from build123d import *

# Parameters (mm, degrees)
F1_DEPTH = 25
F2_R     = 10


with BuildPart() as f1:
    # F0 (on Front) → F1 (new body)
    with BuildSketch(Plane.XZ):
        Polygon((-26.120773, 31.526426), (-26.120773, -33.473574), (12.333255, -33.473574), (32.812056, -19.134163), (23.879227, 31.526426), align=None)
    extrude(amount=F1_DEPTH)

    # F2
    f2_edges = [f1.edges().sort_by_distance(p)[0] for p in [
        (23.879227, -12.5, 31.526426),
        (32.812056, -12.5, -19.134163),
        (-26.120773, -12.5, 31.526426),
        (-26.120773, -12.5, -33.473574),
        (28.345642, -25, 6.196132),
        (-1.120773, -25, 31.526426),
        (-26.120773, -25, -0.973574),
        (-6.893759, -25, -33.473574),
        (22.572655, -25, -26.303868),
        (28.345642, 0, 6.196132),
        (-1.120773, 0, 31.526426),
        (-26.120773, 0, -0.973574),
        (-6.893759, 0, -33.473574),
        (22.572655, 0, -26.303868),
    ]]
    fillet(f2_edges, radius=F2_R)


solid = f1.part
Could you check a few things on this model? Use its own coordinates, in mm. Coordinates: 2 decimals unless noted, no trailing zeros. Write each loop counter-clockwise with the first axis right and the second up, starting at its lowest first coordinate (ties: lowest second). Pieces come first, ordered by that corner, then holes. Notation, with made-up numbers: (9.25, 85.25) - (19.25, 85.25) arc R8 ccw to (19.25, 96.25) - close; hole circle Ø5 at (60, -5). An arc over 180 degrees is marked (long way). Put each result on its own line as item: value. Start each with the question number.
Q1. Thinking about a two-plate mould opening in X: for faces 1 (the flat face through (3, -25, -1)), 2 (the cylindrical face through (-23.27, -3.01, -1.29)), 3 (the flat face through (19.857, -12.465, -28.206)), which applies, pulls with the +X half, pulls with the -X half, needs draft (parallel to the pull), parting line crosses it, or undercut?
Q2. I want a section at B-B on y = -12. Write out the boundary of the cut face in (x, z).
Q3. I want a section at A-A on x = -3. Write out the boundary of the cut face in (y, z).
Q4. I want a section at C-C on z = 27.5. Write out the boundary of the cut face in (x, y), plus the area to 3 significant figures.
Q5. I'm going to push flat-ended pins straight in: P1, Ø6, axis at y = -6, z = 13.5, coming from the +X side; P2, Ø1.5, axis at y = -19, z = 14, coming from the -X side; P3, Ø1, axis at x = 24.5, y = -3.5, coming from the -Z side. Where does each tip first touch, or does it pass through?
Q6. Please list where these lines run through material, in increasing order: L1, parallel to X at y = -21, z = -1.5; L2, parallel to X at y = -11.25, z = -28; L3, parallel to Y at x = 1.5, z = 26.5.
Q7. I want a section at D-D on y = -5.75. Write out the boundary of the cut face in (x, z), plus the area to 3 significant figures.
Checks:
1. face 1: needs draft
1. face 2: pulls with the -X half
1. face 3: pulls with the +X half
2. outline: (-26.12, -23.47) arc R10 ccw to (-16.12, -33.47) - (12.33, -33.47) - (27.59, -22.79) arc R10 ccw to (31.71, -12.86) - (25.34, 23.26) arc R10 ccw to (15.49, 31.53) - (-16.12, 31.53) arc R10 ccw to (-26.12, 21.53) - close
3. outline: (-25, -23.47) arc R10 ccw to (-15, -33.47) - (-10, -33.47) arc R10 ccw to (0, -23.47) - (0, 21.53) arc R10 ccw to (-10, 31.53) - (-15, 31.53) arc R10 ccw to (-25, 21.53) - close
4. outline: (-24.14, -15) arc R8.02 ccw to (-16.12, -23.02) - (15.49, -23.02) arc R8.02 ccw to (23.51, -15) - (23.51, -10) arc R8.02 ccw to (15.49, -1.98) - (-16.12, -1.98) arc R8.02 ccw to (-24.14, -10) - close
4. area: 947 mm²
5. P1: x = 27.25
5. P2: x = -25.58
5. P3: z = -22.63
6. L1: -24.12 to 27.67
6. L2: -25.04 to 20.15
6. L3: -23.68 to -1.32
7. outline: (-25.17, -23.47) arc R9.05 ccw to (-16.12, -32.53) - (12.03, -32.53) - (27.05, -22.01) arc R9.05 ccw to (30.77, -13.02) - (24.4, 23.1) arc R9.05 ccw to (15.49, 30.58) - (-16.12, 30.58) arc R9.05 ccw to (-25.17, 21.53) - close
7. area: 3,190 mm²
